from build123d import *

# Parameters (mm, degrees)
SKETCH_1_W          = 150
SKETCH_1_H          = 60
EXTRUDE_1_DEPTH     = 5
SKETCH_2_R          = 1.55
CUT_EXTRUDE_1_DEPTH = 10
SKETCH_3_R          = 2.05
CUT_EXTRUDE_2_DEPTH = 81.932070281
FILLET_1_R          = 5
CUT_EXTRUDE_3_DEPTH = 10


with BuildPart() as part:
    # 草图1 → 凸台-拉伸1 (new body)
    with BuildSketch(Plane(origin=(0, 0, 0), x_dir=(1, 0, 0), z_dir=(0, 1, 0))):
        Rectangle(SKETCH_1_W, SKETCH_1_H)
    extrude(amount=EXTRUDE_1_DEPTH)

    # 草图2 → 切除-拉伸1 (cut)
    with BuildSketch(Plane(origin=(0, 0, 0), x_dir=(-1, 0, 0), z_dir=(0, -1, 0))):
        with Locations(Location((-66, 20, 0), (0, 0, 90))):
            Circle(SKETCH_2_R)
        with Locations(Location((-42, 20, 0), (0, 0, 90))):
            Circle(SKETCH_2_R)
        with Locations(Location((-66, -10, 0), (0, 0, 90))):
            Circle(SKETCH_2_R)
        with Locations(Location((-42, -10, 0), (0, 0, 90))):
            Circle(SKETCH_2_R)
        with Locations(Location((42, 20, 0), (0, 0, 90))):
            Circle(SKETCH_2_R)
        with Locations(Location((66, 20, 0), (0, 0, 90))):
            Circle(SKETCH_2_R)
        with Locations(Location((42, -10, 0), (0, 0, 90))):
            Circle(SKETCH_2_R)
        with Locations(Location((66, -10, 0), (0, 0, 90))):
            Circle(SKETCH_2_R)
    extrude(amount=-CUT_EXTRUDE_1_DEPTH, mode=Mode.SUBTRACT)

    # 草图3 → 切除-拉伸2 (cut, through all)
    with BuildSketch(Plane(origin=(0, 5, 0), x_dir=(1, 0, 0), z_dir=(0, 1, 0))):
        with Locations(Location((-12, 0, 0), (0, 0, 270))):
            Circle(SKETCH_3_R)
        with Locations(Location((12, 0, 0), (0, 0, 270))):
            Circle(SKETCH_3_R)
        with Locations(Location((-12, -18, 0), (0, 0, 270))):
            Circle(SKETCH_3_R)
        with Locations(Location((12, -18, 0), (0, 0, 270))):
            Circle(SKETCH_3_R)
    extrude(amount=-CUT_EXTRUDE_2_DEPTH, mode=Mode.SUBTRACT)

    # 圆角1
    fillet_1_edges = [part.edges().sort_by_distance(p)[0] for p in [
        (-75, 2.5, -30),
        (75, 2.5, -30),
    ]]
    fillet(fillet_1_edges, radius=FILLET_1_R)

    # 草图4 → 切除-拉伸3 (cut)
    with BuildSketch(Plane(origin=(0, 5, 0), x_dir=(1, 0, 0), z_dir=(0, 1, 0))):
        with BuildLine():
            Line((-50, -15), (-36, -15))
            ThreePointArc((-36, -15), (-31, -20), (-36, -25))
            Line((-36, -25), (-50, -25))
            ThreePointArc((-50, -25), (-55, -20), (-50, -15))
        make_face()
        with BuildLine():
            Line((50, -15), (36, -15))
            ThreePointArc((36, -15), (31, -20), (36, -25))
            Line((36, -25), (50, -25))
            ThreePointArc((50, -25), (55, -20), (50, -15))
        make_face()
    extrude(amount=-CUT_EXTRUDE_3_DEPTH, mode=Mode.SUBTRACT)


solid = part.part
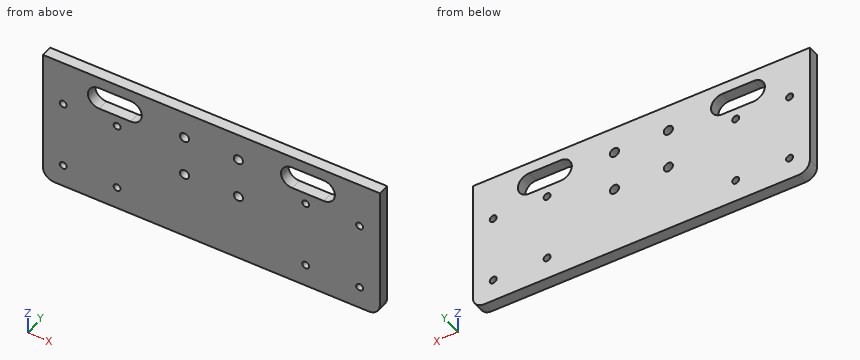
Geometry: final body of the model. Coordinates: model frame, mm. Round coordinates to 2 decimals unless told otherwise and drop trailing zeros. Order: outer loops, then holes, each group sorted by start corner. A loop starts at its lowest first (then second) coordinate and runs counter-clockwise, first axis right, second up.
Q1. Section B-B, the plane x = 42. Output: boundary loops of the cut face in (y, z), and give its area (3 significant figures).
Result sheet:
outline: (0, -30) - (5, -30) - (5, -21.55) - (0, -21.55) - close; (0, -18.45) - (5, -18.45) - (5, 8.45) - (0, 8.45) - close; (0, 11.55) - (5, 11.55) - (5, 15) - (0, 15) - close; (0, 25) - (5, 25) - (5, 30) - (0, 30) - close
area: 219 mm2
Q2. Section D-D, the plane y = 3.55. Give the number of separate pieces and of enclosed holes in the cut face, and give its area (3 significant figures).
Result sheet:
separate pieces: 1
enclosed holes: 14
area: 8,440 mm2
Q3. Section C-C, the plane z = -20. Output: boundary loops of the cut face in (x, y), and give its area (3 significant figures).
Result sheet:
outline: (-75, 0) - (-67.55, 0) - (-67.55, 5) - (-75, 5) - close; (-64.45, 0) - (-43.55, 0) - (-43.55, 5) - (-64.45, 5) - close; (-40.45, 0) - (40.45, 0) - (40.45, 5) - (-40.45, 5) - close; (43.55, 0) - (64.45, 0) - (64.45, 5) - (43.55, 5) - close; (67.55, 0) - (75, 0) - (75, 5) - (67.55, 5) - close
area: 688 mm2
Q4. Pin query (flat end, axial travel): pin 1 (5 mm diameter, centred on x = -66, z = -20, fed in from -Y). Return the tip coordinate at first contact, or that it passes through.
Result sheet:
pin 1: stops at y = 0
Q5. Section A-A, the plane x = -66. Output: boundary loops of the cut face in (y, z).
Result sheet:
outline: (0, -30) - (5, -30) - (5, -21.55) - (0, -21.55) - close; (0, -18.45) - (5, -18.45) - (5, 8.45) - (0, 8.45) - close; (0, 11.55) - (5, 11.55) - (5, 30) - (0, 30) - close
Q6. Material intervals for probe 1 along X at (y, z) = (3.8, 10); probe 2 along Z at (x, y) = (-66, 2.25); probe 3 along Z at (x, y) = (37, 3.6), sorted ascending.
Result sheet:
probe 1: x = -75 to -67.55, -64.45 to -43.55, -40.45 to 40.45, 43.55 to 64.45, 67.55 to 75
probe 2: z = -30 to -21.55, -18.45 to 8.45, 11.55 to 30
probe 3: z = -30 to 15, 25 to 30
